```python
from build123d import *

# Parameters (mm, degrees)
SKETCH_1_R      = 1.55
SKETCH_1_W      = 7.455
SKETCH_1_H      = 13
EXTRUDE_1_DEPTH = 3
FILLET_1_R      = 1


with BuildPart() as part:
    # 草图1 → 凸台-拉伸1 (new body)
    with BuildSketch(Plane.XY):
        with BuildLine():
            Line((-13, 14.5), (-13, 11.5))
            ThreePointArc((-13, 11.5), (-14.005, 10.495), (-15.01, 11.5))
            Line((-15.01, 11.5), (-23.455, 11.5))
            Line((-23.455, 11.5), (-23.455, -11.5))
            Line((-23.455, -11.5), (-15.01, -11.5))
            ThreePointArc((-15.01, -11.5), (-14.005, -10.495), (-13, -11.5))
            Line((-13, -11.5), (-13, -14.5))
            Line((-13, -14.5), (-7, -14.5))
            Line((-7, -14.5), (-7, -11.5))
            ThreePointArc((-7, -11.5), (-5.995, -10.495), (-4.99, -11.5))
            Line((-4.99, -11.5), (23.455, -11.5))
            Line((23.455, -11.5), (23.455, 11.5))
            Line((23.455, 11.5), (-4.99, 11.5))
            ThreePointArc((-4.99, 11.5), (-5.995, 10.495), (-7, 11.5))
            Line((-7, 11.5), (-7, 14.5))
            Line((-7, 14.5), (-13, 14.5))
        make_face()
        with Locations((-20.455, -8)):
            Circle(SKETCH_1_R, mode=Mode.SUBTRACT)
        with Locations((20.455, -8)):
            Circle(SKETCH_1_R, mode=Mode.SUBTRACT)
        Polygon((9.954375568, 0), (7, -4.687005132), (7, 4.687005132), align=None, mode=Mode.SUBTRACT)
        Polygon((11.7275, -2.812994868), (14.681875568, -7.5), (8.773124432, -7.5), align=None, mode=Mode.SUBTRACT)
        with Locations((-12.7275, 0)):
            Rectangle(SKETCH_1_W, SKETCH_1_H, mode=Mode.SUBTRACT)
        with BuildLine():
            Line((-2, -3.5), (-2, -6))
            ThreePointArc((-2, -6), (-3.005, -7.005), (-4.01, -6))
            Line((-4.01, -6), (-5, -6))
            ThreePointArc((-5, -6), (-6.005, -4.995), (-5, -3.99))
            Line((-5, -3.99), (-5, 3.99))
            ThreePointArc((-5, 3.99), (-6.005, 4.995), (-5, 6))
            Line((-5, 6), (-4.01, 6))
            ThreePointArc((-4.01, 6), (-3.005, 7.005), (-2, 6))
            Line((-2, 6), (-2, 3.5))
            Line((-2, 3.5), (4, 3.5))
            Line((4, 3.5), (4, -3.5))
            Line((4, -3.5), (-2, -3.5))
        make_face(mode=Mode.SUBTRACT)
        with Locations((-20.455, 8)):
            Circle(SKETCH_1_R, mode=Mode.SUBTRACT)
        Polygon((16.455, 4.687005132), (16.455, -4.687005132), (13.500624432, 0), align=None, mode=Mode.SUBTRACT)
        Polygon((11.7275, 2.812994868), (8.773124432, 7.5), (14.681875568, 7.5), align=None, mode=Mode.SUBTRACT)
        with Locations((20.455, 8)):
            Circle(SKETCH_1_R, mode=Mode.SUBTRACT)
    extrude(amount=EXTRUDE_1_DEPTH)

    # 圆角1
    fillet_1_edges = [part.edges().sort_by_distance(p)[0] for p in [
        (16.455, -4.687005132, 1.5),
        (16.455, 4.687005132, 1.5),
        (13.500624432, 0, 1.5),
        (14.681875568, -7.5, 1.5),
        (11.7275, -2.812994868, 1.5),
        (8.773124432, -7.5, 1.5),
        (7, 4.687005132, 1.5),
        (7, -4.687005132, 1.5),
        (9.954375568, 0, 1.5),
        (14.681875568, 7.5, 1.5),
        (8.773124432, 7.5, 1.5),
        (11.7275, 2.812994868, 1.5),
    ]]
    fillet(fillet_1_edges, radius=FILLET_1_R)


solid = part.part
```
Check sheet for the modelled part. Datum: model origin and axes. Units: mm. A direction names the side the tool comes from. Coordinates: 2 decimals unless noted, no trailing zeros. Write each loop counter-clockwise with the first axis right and the second up, starting at its lowest first coordinate (ties: lowest second). Pieces come first, ordered by that corner, then holes. Notation, with made-up numbers: M 38,32.5 L 77,32.5 A23 cw 77,59.5 Z; hole C 47.5,63.5 d9. An arc over 180 degrees is marked long. Use one line per item in the form item = value.
Item 1: Release check for a two-part mould opening along X. For faces 3 (the face through (-13, -13, 1)), 4 (the face through (-2, -5, 1)), 5 (the face through (9, 11.5, 1)) record: pulls with the +X half, pulls with the -X half, needs draft (parallel to the pull), parting line crosses it, or undercut.
Answer below:
face_3 = pulls with the -X half
face_4 = undercut
face_5 = needs draft
Item 2: Sectioned sample at D-D, the plane z = 2.2. State how many separate pieces and enclosed holes the cut face has, and give its area (3 significant figures).
Answer below:
separate_pieces = 1
enclosed_holes = 10
area = 855 mm^2
Item 3: Material ranges on L1, parallel to X at y = 3.25, z = 2.6 (3 decimals); L2, parallel to X at y = -5, z = 1 (3 decimals); L3, parallel to Y at x = 1.5, z = 1.5, recorded low to high. Write a range as from..to.
Answer below:
L1 = -23.455..-16.455, -9..-5, 4..23.455
L2 = -23.455..-16.455, -9..-6.005, -2..10.349, 13.106..23.455
L3 = -11.5..-3.5, 3.5..11.5
Item 4: Sectioned sample at C-C, the plane y = -2.75. Record the cut outline in (x, z) (3 decimals), and give its area (3 significant figures).
Answer below:
outline = M -23.455,0 L -16.455,0 L -16.455,3 L -23.455,3 Z; M -9,0 L -5,0 L -5,3 L -9,3 Z; M 4,0 L 23.455,0 L 23.455,3 L 4,3 Z
area = 91.4 mm^2
Item 5: Gauge pin test, flat ends, axial feed: pin 1 Ø1.5 at (x, z) = (8, 1.5) entering from +Y; pin 2 Ø1.5 at (y, z) = (13, 1.5) entering from -X; pin 3 Ø3 at (x, y) = (20.455, 8) entering from -Z; pin 4 Ø0.5 at (x, z) = (-4.5, 1) entering from -Y. Record the tip position at first contact, or that the pin passes through.
Answer below:
pin_1 = 11.5
pin_2 = -13
pin_3 = through
pin_4 = -11.5
Item 6: Set-up check for faces 1 (the face through (13.75, 6.97, 1.52)), 2 (the face through (-10, -14.5, 1)): record each of +Z, -Z, +X, -X, +Y, -Y from which the full face is reachable in a straight line by a thin tool's end or side.
Answer below:
face_1 = +Z, -Z
face_2 = +Z, -Z, +X, -X, -Y
Item 7: Sectioned sample at A-A, the plane y = 8. Record the cut outline in (x, z) (3 decimals).
Answer below:
outline = M -23.455,0 L -22.005,0 L -22.005,3 L -23.455,3 Z; M -18.905,0 L 18.905,0 L 18.905,3 L -18.905,3 Z; M 22.005,0 L 23.455,0 L 23.455,3 L 22.005,3 Z
Item 8: Sectioned sample at B-B, the plane x = -15.5. Record the cut outline in (y, z), and give its area (3 significant figures).
Answer below:
outline = M -11.5,0 L -6.5,0 L -6.5,3 L -11.5,3 Z; M 6.5,0 L 11.5,0 L 11.5,3 L 6.5,3 Z
area = 30.0 mm^2
